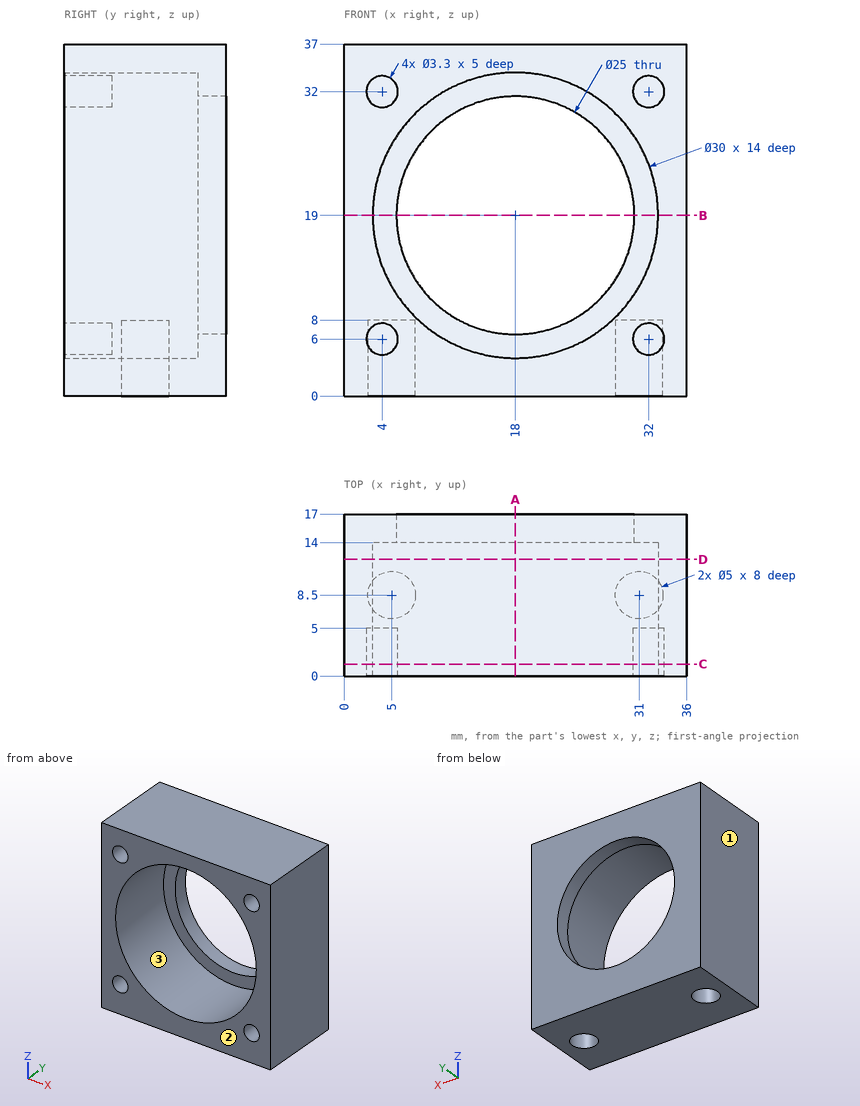
Geometry: see drawing. Coordinates: mm, zero at the bounding-box minimum. Round coordinates to 2 decimals unless told otherwise and drop trailing zeros. Loops run counter-clockwise (first coordinate to the right, second up) from the corner with the lowest first, then second, coordinate; pieces in that order, holes last. Notation, with made-up numbers: (54.5, 30.25) - (92.5, 30.25) arc R29 cw to (92.5, 51.25) - close; hole circle Ø6 at (-32.5, -28). An arc over 180 degrees is marked (long way). Use CSV: the item, a comma, the result in double quotes.
Q1. Section query B-B, the plane z = 19. Output: boundary loops of the cut face in (x, y).
Reported:
outline,"(0, 0) - (3, 0) - (3, 14) - (5.5, 14) - (5.5, 17) - (0, 17) - close; (30.5, 14) - (33, 14) - (33, 0) - (36, 0) - (36, 17) - (30.5, 17) - close"
Q2. Pin query (flat end, axial travel): pin 1 Ø3 at (x, z) = (4, 32) entering from -Y; pin 2 Ø1.5 at (x, y) = (31, 9) entering from -Z; pin 3 Ø15 at (x, z) = (11.5, 19.5) entering from -Y. Return the tip coordinate at first contact, or that it passes through.
Reported:
pin 1,"y = 5"
pin 2,"z = 8"
pin 3,"y = 14"
Q3. Section query C-C, the plane y = 1.25. Output: boundary loops of the cut face in (x, z).
Reported:
outline,"(0, 0) - (36, 0) - (36, 37) - (0, 37) - close; hole circle Ø3.3 at (4, 6); hole circle Ø3.3 at (4, 32); hole circle Ø30 at (18, 19); hole circle Ø3.3 at (32, 6); hole circle Ø3.3 at (32, 32)"
Q4. Mould query, pull axis X, two halves, no side actions, for the marked faces 1, 2 and 3. Classes: pulls with the +X half, pulls with the -X half, needs draft (parallel to the pull), parting line crosses it, or undercut.
Reported:
face 1,"pulls with the -X half"
face 2,"needs draft"
face 3,"undercut"
Q5. Ray query, line 1 along Z through (x, y) = (18, 15.7); line 2 along Y through (x, z) = (5, 1.5); line 3 along X through (y, z) = (5.5, 18.5). Return the intervals inside material, ascending.
Reported:
line 1,"0 to 6.5, 31.5 to 37"
line 2,"0 to 6, 11 to 17"
line 3,"0 to 3.01, 32.99 to 36"
Q6. Section query D-D, the plane y = 12.25. Output: boundary loops of the cut face in (x, z).
Reported:
outline,"(0, 0) - (36, 0) - (36, 37) - (0, 37) - close; hole circle Ø30 at (18, 19)"
Q7. Section query A-A, the plane x = 18. Output: boundary loops of the cut face in (y, z), then the cut area to 3 significant figures.
Reported:
outline,"(0, 0) - (17, 0) - (17, 6.5) - (14, 6.5) - (14, 4) - (0, 4) - close; (0, 34) - (14, 34) - (14, 31.5) - (17, 31.5) - (17, 37) - (0, 37) - close"
area,"134 mm^2"
